```python
from build123d import *

# Parameters (mm, degrees)
F0_W     = 25.4
F0_H     = 41.275
F0_H_2   = 9.525
F0_W_2   = 76.2
F0_W_3   = 4.7625
F0_H_3   = 4.7625
F1_DEPTH = 3.175
F2_R     = 1.27


with BuildPart() as f1:
    # F0 (on Top) → F1 (new body)
    with BuildSketch(Plane.XY):
        with Locations((86.51875, 27.78125)):
            Rectangle(F0_W, F0_H)
        with Locations((86.51875, 2.38125)):
            Rectangle(F0_W, F0_H_2)
        with Locations((35.71875, 2.38125)):
            Rectangle(F0_W_2, F0_H_2)
        with Locations((2.38125, 2.38125)):
            Rectangle(F0_W_3, F0_H_3, mode=Mode.SUBTRACT)
        with Locations((15.08125, 2.38125)):
            Rectangle(F0_W_3, F0_H_3, mode=Mode.SUBTRACT)
        with Locations((27.78125, 2.38125)):
            Rectangle(F0_W_3, F0_H_3, mode=Mode.SUBTRACT)
    extrude(amount=F1_DEPTH)

    # F2
    f2_edges = [f1.edges().sort_by_distance(p)[0] for p in [
        (-2.38125, -2.38125, 1.5875),
        (0, 4.7625, 1.5875),
        (12.7, 4.7625, 1.5875),
        (25.4, 4.7625, 1.5875),
        (-2.38125, 7.14375, 1.5875),
        (0, 0, 1.5875),
        (12.7, 0, 1.5875),
        (25.4, 0, 1.5875),
        (4.7625, 0, 1.5875),
        (17.4625, 0, 1.5875),
        (30.1625, 0, 1.5875),
        (4.7625, 4.7625, 1.5875),
        (17.4625, 4.7625, 1.5875),
        (30.1625, 4.7625, 1.5875),
    ]]
    fillet(f2_edges, radius=F2_R)


solid = f1.part
```
The listing builds one solid part. Answer for the finished solid, in the listing's coordinates (mm). A direction names the side the tool comes from. Coordinates: 2 decimals unless noted, no trailing zeros. Write each loop counter-clockwise with the first axis right and the second up, starting at its lowest first coordinate (ties: lowest second). Pieces come first, ordered by that corner, then holes. Notation, with made-up numbers: (53.5, 20) -> (72.5, 20) arc R27 ccw to (72.5, 45) -> close; hole circle Ø2 at (15, 63). An arc over 180 degrees is marked (long way). Write each question's results on one line, items separated by ' | '. Start each with the question number.
1) A cutting plane is placed at A-A (x = 15). Determine the outline of the cut face in (y, z) (1 decimal), then the cut area to 3 significant figures.
2) A cutting plane is placed at C-C (y = 44). Determine the outline of the cut face in (x, z) (3 decimals), then the cut area to 3 significant figures.
3) A tool of negligible diameter and unlimited length cuts with its end or side. For faces 1 (the flat face through (15, 0, 2)), 2 (the flat face through (70, 6, 0)), 3 (the flat face through (73.819, 28, 2)), from which of +Z, -Z, +X, -X, +Y, -Y can it reach the whole face along a straight path? Write none if from no direction.
4) Straight lines are drawn through the part: probe 1 along X at (y, z) = (3, 0.6); probe 2 along Y at (x, z) = (29, 0.3); probe 3 along Y at (x, z) = (31, 1.6). For each, find the intervals that lie inside material, in ascending order.
5) A cutting plane is placed at B-B (z = 1.3). Count the separate pieces of the cut face and the enclosed holes in it, then the cut area to 3 significant figures.
6) Flat-ended cylindrical pins translate along their axes: pin 1 Ø1.8 at (x, z) = (15.5, 2) entering from +Y; pin 2 Ø1 at (y, z) = (33, 1) entering from -X. Find the tip coordinate at first contact, or state that the pin passes through.
7) For a pull along X with two mould halves and no side action, classify faces 4 (the flat face through (48, -2.381, 2)), 5 (the flat face through (12.7, 2, 2)), 6 (the flat face through (99.219, 23, 2)) as +X half, -X half, draft (parallel to the pull), parting line (faces both ways), or undercut.
Values follow:
1) outline: (-2.4, 0) -> (0, 0) -> (0, 3.2) -> (-2.4, 3.2) -> close; (4.8, 0) -> (7.1, 0) -> (7.1, 3.2) -> (4.8, 3.2) -> close | area: 15.1 mm²
2) outline: (73.819, 0) -> (99.219, 0) -> (99.219, 3.175) -> (73.819, 3.175) -> close | area: 80.6 mm²
3) face 1: +Z, -Z | face 2: -Z, +X, -X, +Y, -Y | face 3: +Z, -Z, -X, +Y
4) probe 1: -2.38 to 0, 4.76 to 12.7, 17.46 to 25.4, 30.16 to 99.22 | probe 2: -2.38 to 0, 4.76 to 7.14 | probe 3: -2.38 to 7.14
5) separate pieces: 1 | enclosed holes: 3 | area: 1,950 mm²
6) pin 1: y = 7.14 | pin 2: x = 73.82
7) face 4: draft | face 5: undercut | face 6: +X half
